Work out the finished part from the listing and answer in its coordinate system (mm). A direction names the side the tool comes from. Round coordinates to 2 decimals unless told otherwise and drop trailing zeros. Loops run counter-clockwise (first coordinate to the right, second up) from the corner with the lowest first, then second, coordinate; pieces in that order, holes last. Notation, with made-up numbers: (28.5, 84) - (32.5, 84) arc R15 cw to (32.5, 104) - close; hole circle Ø3 at (21, 53). An arc over 180 degrees is marked (long way). Return JSON: item names as keys, results as strings.
from build123d import *

# Parameters (mm, degrees)
SKETCH3_R          = 6.35
CUT_EXTRUDE1_DEPTH = 89.9
SHELL1_T           = -1.27
FILLET1_R          = 2.54


with BuildPart() as part:
    # Sketch2 → Revolve1 (revolve)
    with BuildSketch(Plane.XY):
        Polygon((0, 0), (36.195, 0), (22.119166667, 88.9), (0, 88.9), align=None)
    revolve(axis=Axis((0, 88.9, 0), (0, -1, 0)))

    # Sketch3 → Cut-Extrude1 (cut, through all)
    with BuildSketch(Plane.XZ):
        Circle(SKETCH3_R)
    extrude(amount=-CUT_EXTRUDE1_DEPTH, mode=Mode.SUBTRACT)

    # Shell1
    shell1_openings = [part.faces().sort_by_distance(p)[0] for p in [
        (6.35, 0, 0),
    ]]
    offset(amount=SHELL1_T, openings=shell1_openings, kind=Kind.INTERSECTION)

    # Fillet1
    fillet1_edges = [part.edges().sort_by_distance(p)[0] for p in [
        (-7.62, 87.63, 0),
        (-21.034429442, 87.63, 0),
    ]]
    fillet(fillet1_edges, radius=FILLET1_R)


solid = part.part
1) Section A-A (x = 0) is taken. Give the vertices of the cut face in (y, z) (3 decimals), and give its area (3 significant figures).
Verdict:
{"outline": "(0, -36.195) - (88.9, -22.119) - (88.9, -6.35) - (0, -6.35) - (0, -7.62) - (85.09, -7.62) arc R2.54 cw to (87.63, -10.16) - (87.63, -18.865) arc R2.54 cw to (85.487, -21.374) - (0, -34.909) - close; (0, 6.35) - (88.9, 6.35) - (88.9, 22.119) - (0, 36.195) - (0, 34.909) - (85.487, 21.374) arc R2.54 cw to (87.63, 18.865) - (87.63, 10.16) arc R2.54 cw to (85.09, 7.62) - (0, 7.62) - close", "area": "493 mm2"}
2) Section B-B (z = 0) is taken. Give the vertices of the cut face in (x, y) (3 decimals).
Verdict:
{"outline": "(-36.195, 0) - (-34.909, 0) - (-21.374, 85.487) arc R2.54 cw to (-18.865, 87.63) - (-10.16, 87.63) arc R2.54 cw to (-7.62, 85.09) - (-7.62, 0) - (-6.35, 0) - (-6.35, 88.9) - (-22.119, 88.9) - close; (6.35, 0) - (7.62, 0) - (7.62, 85.09) arc R2.54 cw to (10.16, 87.63) - (18.865, 87.63) arc R2.54 cw to (21.374, 85.487) - (34.909, 0) - (36.195, 0) - (22.119, 88.9) - (6.35, 88.9) - close"}
3) Section C-C (y = 64) is taken. Give the vertices of the cut face in (x, z), and give its area (3 significant figures).
Verdict:
{"outline": "circle Ø52.12 at (0, 0); circle Ø15.24 at (0, 0); hole circle Ø49.55 at (0, 0); hole circle Ø12.7 at (0, 0)", "area": "261 mm2"}
4) Find the intervals of material crossed by L1, parallel to Z at x = 0, y = 19; L2, parallel to Z at x = 0, y = 64; L3, parallel to X at y = 51, z = 2.5, in increasing order.
Verdict:
{"L1": "z = -33.19 to -31.9, -7.62 to -6.35, 6.35 to 7.62, 31.9 to 33.19", "L2": "z = -26.06 to -24.78, -7.62 to -6.35, 6.35 to 7.62, 24.78 to 26.06", "L3": "x = -28.01 to -26.72, -7.2 to -5.84, 5.84 to 7.2, 26.72 to 28.01"}
5) Flat-ended cylindrical pins translate along their axes: pin 1 (1.5 mm diameter, centred on y = 70.5, z = 15, fed in from -X); pin 2 (1.5 mm diameter, centred on x = -19, y = 26.5, fed in from -Z); pin 3 (16.5 mm diameter, centred on x = 0, z = 0, fed in from +Y); pin 4 (6 mm diameter, centred on x = -22, y = 68, fed in from +Z). Find the tip coordinate at first contact, or state that the pin passes through.
Verdict:
{"pin 1": "stops at x = -20.6", "pin 2": "stops at z = -26.3", "pin 3": "stops at y = 88.9", "pin 4": "stops at z = 16.97"}
6) Determine the mould class of faces 3 (the flat face through (8, 87.63, -8)), 4 (the conical face through (-6.299, 45.072, -28.368)), 5 (the flat face through (30, 0, 19)) for opening direction Z: pulls with the +Z half, pulls with the -Z half, needs draft (parallel to the pull), parting line crosses it, or undercut.
Verdict:
{"face 3": "undercut", "face 4": "parting line crosses it", "face 5": "needs draft"}
7) Section D-D (y = 21) is taken. Give the vertices of the cut face in (x, z), and give its area (3 significant figures).
Verdict:
{"outline": "circle Ø65.74 at (0, 0); circle Ø15.24 at (0, 0); hole circle Ø63.17 at (0, 0); hole circle Ø12.7 at (0, 0)", "area": "316 mm2"}
8) A tool of negligible diameter and unlimited length cuts with its end or side. For faces 1 (the cylindrical face through (-6.047, 41.949, -4.637)), 2 (the cylindrical face through (-1.38, 43.83, -6.2)), from which of +Z, -Z, +X, -X, +Y, -Y can it reach the whole face along a straight path? Write none if from no direction.
Verdict:
{"face 1": "-Y", "face 2": "+Y, -Y"}
